```python
from build123d import *

# Parameters (mm, degrees)
SKETCH1_W             = 201.5
SKETCH1_H             = 171.5
MAIN_BODY_DEPTH       = 15
SKETCH2_R             = 1.8
SCREW_HOLES_DEPTH     = 15
SKETCH3_R             = 4.15
SKETCH3_R_2           = 1.85
PCB_SCREW_AREA_DEPTH  = 5
SKETCH4_W             = 180
SKETCH4_H             = 150
MAIN_CUT_DEPTH        = 12
FILLET3_R             = 1.2
PCB_START             = -2
SKETCH6_R             = 1.85
PCB_SCREW_HOLES_DEPTH = 2


with BuildPart() as part:
    # Sketch1 → Main Body (new body)
    with BuildSketch(Plane.XY):
        Rectangle(SKETCH1_W, SKETCH1_H)
    extrude(amount=MAIN_BODY_DEPTH)

    # Sketch2 → Screw Holes (cut)
    with BuildSketch(Plane.XY.offset(15)):
        with Locations((-97.5, 82.5)):
            Circle(SKETCH2_R)
        with Locations((97.5, 82.5)):
            Circle(SKETCH2_R)
        with Locations((97.5, -82.5)):
            Circle(SKETCH2_R)
        with Locations((-97.5, -82.5)):
            Circle(SKETCH2_R)
    extrude(amount=-SCREW_HOLES_DEPTH, mode=Mode.SUBTRACT)

    # Sketch3 → PCB Screw Area (add)
    # profile 1 of 4: a face of its own
    with BuildSketch(Plane.XY.offset(15)):
        with Locations((-37.7639992, -17.5345021)):
            Circle(SKETCH3_R)
        with Locations((-37.7639992, -17.5345021)):
            Circle(SKETCH3_R_2, mode=Mode.SUBTRACT)
    # profile 2 of 4: a face of its own
    with BuildSketch(Plane.XY.offset(15)):
        with Locations((54.6920008, -17.5345021)):
            Circle(SKETCH3_R)
        with Locations((54.6920008, -17.5345021)):
            Circle(SKETCH3_R_2, mode=Mode.SUBTRACT)
    # profile 3 of 4: a face of its own
    with BuildSketch(Plane.XY.offset(15)):
        with Locations((54.5650008, -70.7475021)):
            Circle(SKETCH3_R)
        with Locations((54.5650008, -70.7475021)):
            Circle(SKETCH3_R_2, mode=Mode.SUBTRACT)
    # profile 4 of 4: a face of its own
    with BuildSketch(Plane.XY.offset(15)):
        with Locations((-38.3989992, -70.7475021)):
            Circle(SKETCH3_R)
        with Locations((-38.3989992, -70.7475021)):
            Circle(SKETCH3_R_2, mode=Mode.SUBTRACT)
    extrude(amount=PCB_SCREW_AREA_DEPTH)

    # Sketch4 → Main Cut (cut)
    with BuildSketch(Plane(origin=(0, 0, 0), x_dir=(-1, 0, 0), z_dir=(0, 0, -1))):
        Rectangle(SKETCH4_W, SKETCH4_H)
    extrude(amount=-MAIN_CUT_DEPTH, mode=Mode.SUBTRACT)

    # Fillet3
    fillet3_edges = [part.edges().sort_by_distance(p)[0] for p in [
        (-42.5489992, -70.7475021, 15),
        (50.4150008, -70.7475021, 15),
        (50.5420008, -17.5345021, 15),
        (-41.9139992, -17.5345021, 15),
    ]]
    fillet(fillet3_edges, radius=FILLET3_R)

    # Sketch6 → PCB Screw Holes (cut)
    with BuildSketch(Plane.XY.offset(15).offset(PCB_START)):
        with Locations((-37.7639992, -17.5345021)):
            Circle(SKETCH6_R)
        with Locations((-38.3989992, -70.7475021)):
            Circle(SKETCH6_R)
        with Locations((54.5650008, -70.7475021)):
            Circle(SKETCH6_R)
        with Locations((54.6920008, -17.5345021)):
            Circle(SKETCH6_R)
    extrude(amount=PCB_SCREW_HOLES_DEPTH, mode=Mode.SUBTRACT)


solid = part.part
```
Input: part model. Units: mm. Frame: model coordinates. A direction names the side the tool comes from. Coordinates: 2 decimals unless noted, no trailing zeros. Loops run counter-clockwise (first coordinate to the right, second up) from the corner with the lowest first, then second, coordinate; pieces in that order, holes last. Notation, with made-up numbers: (48, -28) -> (103, -28) arc R32 cw to (103, 8) -> close; hole circle Ø9 at (79.25, 37). An arc over 180 degrees is marked (long way). Use a Markdown table: item, result.
1) Material intervals for line 1 along X through (y, z) = (-82.5, 9); line 2 along Y through (x, z) = (97.5, 3.75); line 3 along Y through (x, z) = (-12.5, 2.25), sorted ascending. Write a range as from..to.
Results found:
| item | result |
|---|---|
| line 1 | x = -100.75..-99.3, -95.7..95.7, 99.3..100.75 |
| line 2 | y = -85.75..-84.3, -80.7..80.7, 84.3..85.75 |
| line 3 | y = -85.75..-75, 75..85.75 |
2) Cut plane C-C (x = -65.5). Return the cut outline in (y, z).
Results found:
| item | result |
|---|---|
| outline | (-85.75, 0) -> (-75, 0) -> (-75, 12) -> (75, 12) -> (75, 0) -> (85.75, 0) -> (85.75, 15) -> (-85.75, 15) -> close |
3) Cut plane B-B (z = 5.5). Return the cut outline in (x, y).
Results found:
| item | result |
|---|---|
| outline | (-100.75, -85.75) -> (100.75, -85.75) -> (100.75, 85.75) -> (-100.75, 85.75) -> close; hole circle Ø3.6 at (-97.5, -82.5); hole circle Ø3.6 at (-97.5, 82.5); hole (-90, -75) -> (90, -75) -> (90, 75) -> (-90, 75) -> close; hole circle Ø3.6 at (97.5, -82.5); hole circle Ø3.6 at (97.5, 82.5) |
4) Contact query for flat-ended pins moving along their axis: pin 1 (3.5 mm diameter, centred on x = -38.4, y = -70.75, fed in from -Z); pin 2 (1 mm diameter, centred on x = 76.5, y = -14.5, fed in from +Z); pin 3 (1.1 mm diameter, centred on x = 54, y = -71.5, fed in from +Z). Output: stop coordinate, or through.
Results found:
| item | result |
|---|---|
| pin 1 | stops at z = 12 |
| pin 2 | stops at z = 15 |
| pin 3 | stops at z = 13 |
5) Cut plane A-A (y = 11). Return the cut outline in (x, z), then the cut area to 4 significant figures.
Results found:
| item | result |
|---|---|
| outline | (-100.75, 0) -> (-90, 0) -> (-90, 12) -> (90, 12) -> (90, 0) -> (100.75, 0) -> (100.75, 15) -> (-100.75, 15) -> close |
| area | 862.5 mm2 |
6) Access query for faces 1 (the cylindrical face through (54.025, -66.633, 18.073)), 2 (the flat face through (-90, -1, 6)), 3 (the flat face through (-1, -85.75, 7)). Directions: +Z, -Z, +X, -X, +Y, -Y. A direction counts if a zero-diameter tool reaches every point of the face in a straight line with its end or side. Return the directions, or none.
Results found:
| item | result |
|---|---|
| face 1 | +Z |
| face 2 | -Z |
| face 3 | +Z, -Z, +X, -X, -Y |
